from build123d import *

# Parameters (mm, degrees)
F1_DEPTH = 78.3572047949
F2_R     = 38.5370833617
F3_DEPTH = 25.4
F5_W     = 13.0668841302
F5_H     = 27.1093435585
F5_W_2   = 25.3738258034
F5_H_2   = 12.5543624163
F6_DEPTH = 5.4576825351


with BuildPart() as f1:
    # F0 (on Front) → F1 (new body)
    with BuildSketch(Plane.XZ):
        with BuildLine():
            ThreePointArc((0, 42.2524884343), (-29.8770210939, -29.8770210939), (42.2524884343, 0))
            ThreePointArc((42.2524884343, 0), (29.8770210939, 29.8770210939), (0, 42.2524884343))
        make_face()
    extrude(amount=F1_DEPTH)

    # F2 (on face) → F3 (cut)
    with BuildSketch(Plane.XZ.offset(78.3572047949)):
        Circle(F2_R)
    extrude(amount=-F3_DEPTH, mode=Mode.SUBTRACT)

    # F5 (on face) → F6 (join)
    with BuildSketch(Plane(origin=(0, 0, 0), x_dir=(-1, 0, 0), z_dir=(0, 1, 0))):
        with Locations((0, 19.8318529874)):
            Rectangle(F5_W, F5_H)
        with Locations((19.2203549668, 0)):
            Rectangle(F5_W_2, F5_H_2)
        with Locations((0, -19.8318529874)):
            Rectangle(F5_W, F5_H)
        with Locations((-19.2203549668, 0)):
            Rectangle(F5_W_2, F5_H_2)
        Rectangle(F5_W, F5_H_2)
    extrude(amount=F6_DEPTH)


solid = f1.part
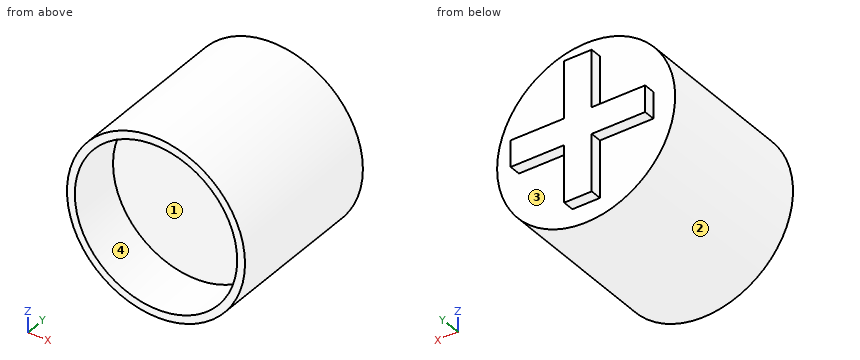
Can you work these out from the model? Positions are in its coordinate system, mm. Face numbers are marked on the shaded views. Coordinates: 2 decimals unless noted, no trailing zeros. Write each loop counter-clockwise with the first axis right and the second up, starting at its lowest first coordinate (ties: lowest second). Pieces come first, ordered by that corner, then holes. Notation, with made-up numbers: (87.5, 14) - (94.5, 14) arc R18 ccw to (94.5, 35) - close; hole circle Ø11 at (77.25, 66.5). An arc over 180 degrees is marked (long way). Return JSON: item names as keys, results as strings. Group by question number.
Item 1: If we section it at A-A (x = 0): Write out the boundary of the cut face in (y, z), then the cut area to 3 significant figures.
Item 2: Please list where these lines run through material, in increasing order: probe 1 along Z at (x, y) = (0, -65.25); probe 2 along X at (y, z) = (-36.5, 1.5); probe 3 along Y at (x, z) = (-1.5, -22.5).
Item 3: If we section it at D-D (y = -18.5): Write out the boundary of the cut face in (x, z).
Item 4: We'd pull the mould along Z, two halves only. Please class the marked faces 1, 2, 3 and 4: pulls with the +Z half, pulls with the -Z half, needs draft (parallel to the pull), parting line crosses it, or undercut.
Item 5: If we section it at B-B (z = 0): Write out the boundary of the cut face in (x, y), then the cut area to 3 significant figures.
Item 6: I'm going to push flat-ended pins straight in: pin 1 Ø2.5 at (y, z) = (3, -2.5) entering from +X; pin 2 Ø3 at (x, y) = (20, -39) entering from -Z; pin 3 Ø4 at (x, z) = (-9.5, -10.5) entering from -Y. Where does each tip first touch, or does it pass through?
Item 7: If we section it at C-C (y = -67): Write out the boundary of the cut face in (x, z).
Return value:
{
 "1": {"outline": "(-78.36, -42.25) - (0, -42.25) - (0, -33.39) - (5.46, -33.39) - (5.46, 33.39) - (0, 33.39) - (0, 42.25) - (-78.36, 42.25) - (-78.36, 38.54) - (-52.96, 38.54) - (-52.96, -38.54) - (-78.36, -38.54) - close", "area": "5,030 mm^2"},
 "2": {"probe 1": "z = -42.25 to -38.54, 38.54 to 42.25", "probe 2": "x = -42.23 to 42.23", "probe 3": "y = -52.96 to 5.46"},
 "3": {"outline": "circle Ø84.5 at (0, 0)"},
 "4": {"face 1": "undercut", "face 2": "parting line crosses it", "face 3": "needs draft", "face 4": "undercut"},
 "5": {"outline": "(-42.25, -78.36) - (-38.54, -78.36) - (-38.54, -52.96) - (38.54, -52.96) - (38.54, -78.36) - (42.25, -78.36) - (42.25, 0) - (31.91, 0) - (31.91, 5.46) - (-31.91, 5.46) - (-31.91, 0) - (-42.25, 0) - close", "area": "5,010 mm^2"},
 "6": {"pin 1": "stops at x = 31.91", "pin 2": "stops at z = -37.99", "pin 3": "stops at y = -52.96"},
 "7": {"outline": "circle Ø84.5 at (0, 0); hole circle Ø77.07 at (0, 0)"}
}
